Source: CAD feature listing. Evaluate the final solid. Frame: model axes, mm. A direction names the side the tool comes from. Round coordinates to 2 decimals unless told otherwise and drop trailing zeros.
from build123d import *

# Parameters (mm, degrees)
SKETCH_W          = 25
SKETCH_H          = 25
PAD_DEPTH         = 15
SKETCH002_W       = 21
SKETCH002_H       = 21
SKETCH001_W       = 23
SKETCH001_H       = 23
SKETCH004_W       = 25
SKETCH004_H       = 25
PAD001_DEPTH      = 20
BOX_W             = 20
BOX_H             = 20
BOX_DEPTH         = 21
BOX001_W          = 5
BOX001_H          = 5
BOX001_DEPTH      = 5
BOX002_W          = 5
BOX002_H          = 5
BOX002_DEPTH      = 5
BOX003_W          = 5
BOX003_H          = 5
BOX003_DEPTH      = 5
BOX004_W          = 5
BOX004_H          = 5
BOX004_DEPTH      = 5
CYLINDER_R        = 1.5
CYLINDER_DEPTH    = 10
CYLINDER001_R     = 1.5
CYLINDER001_DEPTH = 10
CYLINDER002_R     = 1.5
CYLINDER002_DEPTH = 10
CYLINDER003_R     = 1.5
CYLINDER003_DEPTH = 13


with BuildPart() as body:
    # Sketch → Pad (new body)
    with BuildSketch(Plane.XY):
        Rectangle(SKETCH_W, SKETCH_H)
    extrude(amount=PAD_DEPTH)

    # Sketch002 (on Face5 of Pad) → SubtractiveLoft section 0
    with BuildSketch(Plane(origin=(0, 0, 0), x_dir=(1, 0, 0), z_dir=(0, 0, -1))):
        Rectangle(SKETCH002_W, SKETCH002_H)
    # Sketch001 (on Face6 of Pad) → SubtractiveLoft section 1
    with BuildSketch(Plane.XY.offset(15)):
        Rectangle(SKETCH001_W, SKETCH001_H)
    loft(mode=Mode.SUBTRACT)


with BuildPart() as body001:
    # Sketch004 → Pad001 (new body)
    with BuildSketch(Plane.XY):
        Rectangle(SKETCH004_W, SKETCH004_H)
    extrude(amount=PAD001_DEPTH)

    # Boolean: cut Body
    add(body.part, mode=Mode.SUBTRACT)

    # Box → Box (cut)
    with BuildSketch(Plane(origin=(-10, -10, 0), x_dir=(1, 0, 0), z_dir=(0, 0, 1))):
        with Locations((10, 10)):
            Rectangle(BOX_W, BOX_H)
    extrude(amount=BOX_DEPTH, mode=Mode.SUBTRACT)

    # Box001 → Box001 (join)
    with BuildSketch(Plane(origin=(-10, 10, 0), x_dir=(1, 0, 0), z_dir=(0, -1, 0))):
        with Locations((2.5, 2.5)):
            Rectangle(BOX001_W, BOX001_H)
    extrude(amount=BOX001_DEPTH)

    # Box002 → Box002 (join)
    with BuildSketch(Plane(origin=(10, 10, 5), x_dir=(0, 0, -1), z_dir=(-1, 0, 0))):
        with Locations((2.5, 2.5)):
            Rectangle(BOX002_W, BOX002_H)
    extrude(amount=BOX002_DEPTH)

    # Box003 → Box003 (join)
    with BuildSketch(Plane(origin=(10, -10, 5), x_dir=(0, 0, -1), z_dir=(0, 1, 0))):
        with Locations((2.5, 2.5)):
            Rectangle(BOX003_W, BOX003_H)
    extrude(amount=BOX003_DEPTH)

    # Box004 → Box004 (join)
    with BuildSketch(Plane(origin=(-10, -10, 5), x_dir=(0, 0, -1), z_dir=(1, 0, 0))):
        with Locations((2.5, 2.5)):
            Rectangle(BOX004_W, BOX004_H)
    extrude(amount=BOX004_DEPTH)

    # Cylinder → Cylinder (cut)
    with BuildSketch(Plane(origin=(-7.5, 7.5, -1.5), x_dir=(0, -1, 0), z_dir=(0, 0, 1))):
        Circle(CYLINDER_R)
    extrude(amount=CYLINDER_DEPTH, mode=Mode.SUBTRACT)

    # Cylinder001 → Cylinder001 (cut)
    with BuildSketch(Plane(origin=(7.5, 7.5, -3), x_dir=(0, -1, 0), z_dir=(0, 0, 1))):
        Circle(CYLINDER001_R)
    extrude(amount=CYLINDER001_DEPTH, mode=Mode.SUBTRACT)

    # Cylinder002 → Cylinder002 (cut)
    with BuildSketch(Plane(origin=(7.5, -7.5, -4), x_dir=(0, -1, 0), z_dir=(0, 0, 1))):
        Circle(CYLINDER002_R)
    extrude(amount=CYLINDER002_DEPTH, mode=Mode.SUBTRACT)

    # Cylinder003 → Cylinder003 (cut)
    with BuildSketch(Plane(origin=(-7.5, -7.5, -8), x_dir=(0, -1, 0), z_dir=(0, 0, 1))):
        Circle(CYLINDER003_R)
    extrude(amount=CYLINDER003_DEPTH, mode=Mode.SUBTRACT)


solid = body001.part
1) Section query A-A on y = 7.5. State how many separate pieces and enclosed holes the cut face has, then the cut area to 3 significant figures.
Taken from the geometry:
separate pieces: 4
enclosed holes: 0
area: 75.0 mm2
2) Contact query for flat-ended pins moving along their axis: P1, Ø2, axis at x = 5, z = 7.5, coming from the -Y side; P2, Ø2, axis at x = 0, z = 6, coming from the +Y side; P3, Ø4, axis at x = -7.5, y = -7, coming from the +Z side; P4, Ø1.5, axis at x = 8, y = 8, coming from the +Z side. Output: stop coordinate, or through.
Taken from the geometry:
P1: stops at y = -11.07
P2: stops at y = 10.97
P3: stops at z = 5
P4: passes through
3) Material intervals for line 1 (X direction, y = -3.75, z = 16.5); line 2 (X direction, y = 7.5, z = 2.05); line 3 (Y direction, x = 7.5, z = 2.9), sorted ascending.
Taken from the geometry:
line 1: x = -12.5 to -10, 10 to 12.5
line 2: x = -10.64 to -9, -6 to -5, 5 to 6, 9 to 10.64
line 3: y = -10.69 to -9, -6 to -5, 5 to 6, 9 to 10.69
4) Pull-direction query (X, two-part tool) for faces 1 (the face through (12.5, 0, 17)), 2 (the face through (0, 12.5, 17)), 3 (the face through (-8, 5, 3)); classes: released by +X, released by -X, zero draft, split by the parting line, or undercut.
Taken from the geometry:
face 1: released by +X
face 2: zero draft
face 3: undercut
5) Reachability of faces 4 (the face through (0, 10, 10)), 5 (the face through (5, 7, 3)), 6 (the face through (5.4, -5.4, 0)), 7 (the face through (0, -12.5, 17)), 8 (the face through (-1, -12, 15)) from +Z, -Z, +X, -X, +Y, -Y: full face, straight path, thin tool, end or side. Return the list, or none.
Taken from the geometry:
face 4: +Z
face 5: +Z, -Z
face 6: -Z, +X, -X, +Y, -Y
face 7: +Z, -Z, +X, -X, -Y
face 8: -Z
